Geometry check sheet. Reference: the model listing, model coordinates, mm. A direction names the side the tool comes from. Give positions to 0.01 mm unless a question says otherwise; leave off trailing zeros. Write each loop counter-clockwise with the first axis right and the second up, starting at its lowest first coordinate (ties: lowest second). Pieces come first, ordered by that corner, then holes. Notation, with made-up numbers: (56.25, -28) -> (115.25, -28) arc R10 cw to (115.25, -14) -> close; hole circle Ø1 at (8.25, 47.25). An arc over 180 degrees is marked (long way). Use a Markdown table: item, result. Add a question column.
Autodesk Inventor part; units mm, degrees
ref_plane "作業平面1" through (0, 6, 0) normal (0, 1, 0) x (-1, 0, 0)
ref_plane "YZ Plane" through (0, 0, 0) normal (1, 0, 0) x (0, 1, 0)
ref_plane "XY Plane" through (0, 0, 0) normal (0, 0, 1) x (1, 0, 0)
sketch "スケッチ1" plane through (0, 0, 0) normal (0, 0, 1) x (1, 0, 0)
  circle A0 centre (0, 0) radius 6
  dimension "d0" = 12
extrude "押し出し1" add sketch "スケッチ1" along normal blind 50
ref_plane "作業平面1" through (0, 6, 0) normal (0, 1, 0) x (-1, 0, 0)
sketch "スケッチ2" plane through (0, 6, 0) normal (0, 1, 0) x (-1, 0, 0)
  line L0 (0, 0) -> (2, 0)
  line L1 (2, 0) -> (2, 20)
  line L2 (2, 20) -> (0, 20)
  line L3 (0, 20) -> (0, 0)
  line L4 (6, 0) -> (-6, 0)
  line L5 (0, 20) -> (-2, 20)
  line L6 (-2, 20) -> (-2, 0)
  line L7 (-2, 0) -> (0, 0)
  line L8 (0, 0) -> (0, 20)
  dimension "d3" = 2
  dimension "d4" = 20
  dimension "d5" = 2
extrude "押し出し2" cut sketch "スケッチ2" against normal blind 6
sketch "スケッチ3" plane through (0, 0, 0) normal (0, 0, -1) x (-1, 0, 0)
  point P0 (0, 0)
  point P1 (0, 0)
hole "穴1" at (0, 0, 0) direction (0, 0, 1) diameter 8 depth 20 tip angle 118
sketch "スケッチ4" plane through (0, 6, 0) normal (0, 1, 0) x (-1, 0, 0)
  line L0 (2, 20) -> (-2, 20)
  point P0 (0, 0)
  point P1 (0, 35)
  dimension "d15" = 15
hole "穴2" at (0, 6, 35) direction (0, -1, 0) diameter 4 end through all
sketch "スケッチ5" plane through (0, 6, 0) normal (0, 1, 0) x (-1, 0, 0)
  line L0 (6, 50) -> (-6, 50)
  point P0 (0, 0)
  point P1 (0, 47)
  dimension "d23" = 3
hole "穴3" at (0, 6, 47) direction (0, -1, 0) diameter 2 end through all
properties part number "jik_motor_10-50" material "アルミニウム 6061-AHC"
1) Sectioned sample at D-D, the plane x = -4.5. Enter the section's corners in (y, z), and give its area (3 significant figures).
2) Sectioned sample at C-C, the plane y = 2.25. Count the separate pieces of the cut face and the enclosed holes in it, and give its area (3 significant figures).
3) Sectioned sample at A-A, the plane z = 35. Enter the section's corners in (x, y), and give its area (3 significant figures).
4) Material ranges on probe 1 along Z at (x, y) = (-0.75, 2); probe 2 along Z at (x, y) = (0, 1); probe 3 along X at (y, z) = (0, 35), recorded low to high. Write a range as [from, to].
5) Tool access check on faces 4 (the face through (-2, 5, 10)), 5 (the face through (0, -4, 10)), 6 (the face through (0.766, -0.084, 36.847)). Record the directions out of +Z, -Z, +X, -X, +Y, -Y that give a thin tool (end or side, any length) a straight path to the whole face; none if there is none.
6) Draft check along X on faces 1 (the face through (1.2, -4, 0)), 2 (the face through (3.226, -5.059, 24.65)), 3 (the face through (2, 5, 10)). Enter one of: +X half, -X half, draft (parallel to the pull), parting line (faces both ways), or undercut.
7) Sectioned sample at B-B, the plane z = 29. Enter the section's corners in (x, y), and give its area (3 significant figures).
8) Gauge pin test, flat ends, axial feed: P1, Ø1.5, axis at x = -1, y = -2.5, coming from the -Z side; P2, Ø2.5, axis at y = 4, z = 11.5, coming from the -X side; P3, Ø0.8, axis at x = -0.5, y = 5.5, coming from the -Z side. Record the tip position at first contact, or that the pin passes through.
Check values:
| question | item | result |
|---|---|---|
| 1 | outline | (-3.97, 0) -> (3.97, 0) -> (3.97, 50) -> (-3.97, 50) -> close |
| 1 | area | 397 mm² |
| 2 | separate pieces | 1 |
| 2 | enclosed holes | 2 |
| 2 | area | 404 mm² |
| 3 | outline | (-2, -5.66) -> (-2, 5.66) arc R6 ccw to start; (2, -5.66) arc R6 ccw to (2, 5.66) -> close |
| 3 | area | 66.0 mm² |
| 4 | probe 1 | [21.12, 33.15], [36.85, 46.34], [47.66, 50] |
| 4 | probe 2 | [21.8, 33], [37, 46], [48, 50] |
| 4 | probe 3 | [-6, -2], [2, 6] |
| 5 | face 4 | -Z, +Y |
| 5 | face 5 | -Z |
| 5 | face 6 | +Y, -Y |
| 6 | face 1 | draft |
| 6 | face 2 | parting line |
| 6 | face 3 | undercut |
| 7 | outline | circle Ø12 at (0, 0) |
| 7 | area | 113 mm² |
| 8 | P1 | z = 20.33 |
| 8 | P2 | x = -5.33 |
| 8 | P3 | z = 20 |
